from build123d import *

# Parameters (mm, degrees)
F0_W     = 81.72
F0_H     = 134.06
F1_DEPTH = 13.04
F2_W     = 81.72
F2_H     = 60.06
F3_DEPTH = 3.12
F4_W     = 81.72
F4_H     = 68.02
F5_DEPTH = 3.12
F6_R     = 5.72
F7_DEPTH = 25.4
F9_DEPTH = 25.4
F10_R    = 12.7


with BuildPart() as f1:
    # F0 (on Top) → F1 (new body)
    with BuildSketch(Plane.XY):
        Rectangle(F0_W, F0_H)
    extrude(amount=F1_DEPTH)

    # F2 (on face) → F3 (join)
    with BuildSketch(Plane.XY.offset(13.04)):
        Rectangle(F2_W, F2_H)
    extrude(amount=F3_DEPTH)

    # F4 (on face) → F5 (cut)
    with BuildSketch(Plane(origin=(0, 0, 0), x_dir=(1, 0, 0), z_dir=(0, 0, -1))):
        Rectangle(F4_W, F4_H)
    extrude(amount=-F5_DEPTH, mode=Mode.SUBTRACT)

    # F6 (on face) → F7 (cut)
    with BuildSketch(Plane.XY.offset(13.04)):
        with Locations((-27.55223, 53.701179)):
            Circle(F6_R)
        with Locations((27.534222, 53.702354)):
            Circle(F6_R)
    extrude(amount=-F7_DEPTH, mode=Mode.SUBTRACT)

    # F8 (on face) → F9 (cut)
    with BuildSketch(Plane.XY.offset(13.04)):
        with BuildLine():
            ThreePointArc((-27.53, -59.42), (-23.485349, -57.744651), (-21.81, -53.7))
            ThreePointArc((-21.81, -53.7), (-27.53, -47.98), (-33.25, -53.7))
            ThreePointArc((-33.25, -53.7), (-31.574651, -57.744651), (-27.53, -59.42))
        make_face()
        with BuildLine():
            ThreePointArc((27.53, -59.42), (31.574651, -57.744651), (33.25, -53.7))
            ThreePointArc((33.25, -53.7), (23.485349, -49.655349), (27.53, -59.42))
        make_face()
    extrude(amount=-F9_DEPTH, mode=Mode.SUBTRACT)

    # F10
    f10_edges = [f1.edges().sort_by_distance(p)[0] for p in [
        (-40.86, 67.03, 6.52),
        (40.86, 67.03, 6.52),
        (40.86, -67.03, 6.52),
        (-40.86, -67.03, 6.52),
    ]]
    fillet(f10_edges, radius=F10_R)


solid = f1.part
Design review of the part built by this model. Coordinates are the model's own, in mm. A direction names the side the tool comes from. Round coordinates to 2 decimals unless told otherwise and drop trailing zeros. Write each loop counter-clockwise with the first axis right and the second up, starting at its lowest first coordinate (ties: lowest second). Pieces come first, ordered by that corner, then holes. Notation, with made-up numbers: (33, -18) - (91, -18) arc R30 cw to (91, 11) - close; hole circle Ø4 at (3, 83). An arc over 180 degrees is marked (long way). Use a Markdown table: item, result. Add a question column.
1. We need section B-B (x = 15.5). State the section outline as (y, z) points, then the cut area to 3 significant figures.
2. We need section C-C (y = 23.5). State the section outline as (x, z) points.
3. We need section D-D (z = 9). State the section outline as (x, y) points.
4. Mouldability with a two-part tool opening along X and no side actions: class faces 1 (the face through (-24.91, 48.63, 6.61)), 2 (the face through (-40.86, -1, 8)), 3 (the face through (-1, 30.03, 15)) as +X half, -X half, draft (parallel to the pull), parting line (faces both ways), or undercut.
5. Clearance check with flat-ended pins moving along their axes: pin 1 (18.5 mm diameter, centred on x = 27.53, y = -53.7, fed in from +Z); pin 2 (2.5 mm diameter, centred on x = -14.5, z = 15, fed in from +Y); pin 3 (5 mm diameter, centred on x = -32, z = 5.5, fed in from +Y). State where each tip first meets the part, or that it passes through.
6. For faces 4 (the face through (-1, 34.01, 2)), 5 (the face through (-1, 49, 13.04)), 6 (the face through (-1, -30.03, 15)), 7 (the face through (-1, 0, 16.16)), list the 3-axis set-ups (+Z, -Z, +X, -X, +Y, -Y) from which the entire face can be reached by the end or side of a thin tool; tool diameter is ignored.
7. Wall thickness on probe 1 along X at (y, z) = (-53.7, 5.5); probe 2 along Y at (x, z) = (27.53, 6.75); probe 3 along Y at (x, z) = (-26, 8): over which ranges is each line inside the solid? List them lowest first.
8. We need section A-A (z = 1.75). State the section outline as (x, y) points, then the cut area to 3 significant figures.
Output:
| question | item | result |
|---|---|---|
| 1 | outline | (-67.03, 0) - (-34.01, 0) - (-34.01, 3.12) - (34.01, 3.12) - (34.01, 0) - (67.03, 0) - (67.03, 13.04) - (30.03, 13.04) - (30.03, 16.16) - (-30.03, 16.16) - (-30.03, 13.04) - (-67.03, 13.04) - close |
| 1 | area | 1,720 mm2 |
| 2 | outline | (-40.86, 3.12) - (40.86, 3.12) - (40.86, 16.16) - (-40.86, 16.16) - close |
| 3 | outline | (-40.86, -54.33) arc R12.7 ccw to (-28.16, -67.03) - (28.16, -67.03) arc R12.7 ccw to (40.86, -54.33) - (40.86, 54.33) arc R12.7 ccw to (28.16, 67.03) - (-28.16, 67.03) arc R12.7 ccw to (-40.86, 54.33) - close; hole circle Ø11.44 at (-27.55, 53.7); hole circle Ø11.44 at (-27.53, -53.7); hole circle Ø11.44 at (27.53, -53.7); hole circle Ø11.44 at (27.53, 53.7) |
| 4 | face 1 | undercut |
| 4 | face 2 | -X half |
| 4 | face 3 | draft |
| 5 | pin 1 | stops at z = 13.04 |
| 5 | pin 2 | stops at y = 30.03 |
| 5 | pin 3 | stops at y = 66.96 |
| 6 | face 4 | -Z, +X, -X |
| 6 | face 5 | +Z, +X, -X, +Y |
| 6 | face 6 | +Z, +X, -X, -Y |
| 6 | face 7 | +Z, +X, -X, +Y, -Y |
| 7 | probe 1 | x = -40.86 to -33.25, -21.81 to 21.81, 33.25 to 40.86 |
| 7 | probe 2 | y = -67.03 to -59.42, -47.98 to 47.98, 59.42 to 67.03 |
| 7 | probe 3 | y = -67.03 to -59.21, -48.19 to 48.2, 59.21 to 67.03 |
| 8 | outline | (-40.86, -54.33) arc R12.7 ccw to (-28.16, -67.03) - (28.16, -67.03) arc R12.7 ccw to (40.86, -54.33) - (40.86, -34.01) - (-40.86, -34.01) - close; (-40.86, 34.01) - (40.86, 34.01) - (40.86, 54.33) arc R12.7 ccw to (28.16, 67.03) - (-28.16, 67.03) arc R12.7 ccw to (-40.86, 54.33) - close; hole circle Ø11.44 at (-27.55, 53.7); hole circle Ø11.44 at (-27.53, -53.7); hole circle Ø11.44 at (27.53, -53.7); hole circle Ø11.44 at (27.53, 53.7) |
| 8 | area | 4,850 mm2 |
